Here's the drawing with two shaded views (mm, measured from the low corner). I have some questions. Give positions to 0.01 mm unless a question says otherwise; leave off trailing zeros. Order: outer loops, then holes, each group sorted by start corner. A loop starts at its lowest first (then second) coordinate and runs counter-clockwise, first axis right, second up. Notation, with made-up numbers: M -0.5,86.5 L 43.5,86.5 A14 ccw 43.5,106.5 Z; hole C 22,74.5 d8. An arc over 180 degrees is marked long. Use a Markdown table: item, result. Add a question column.
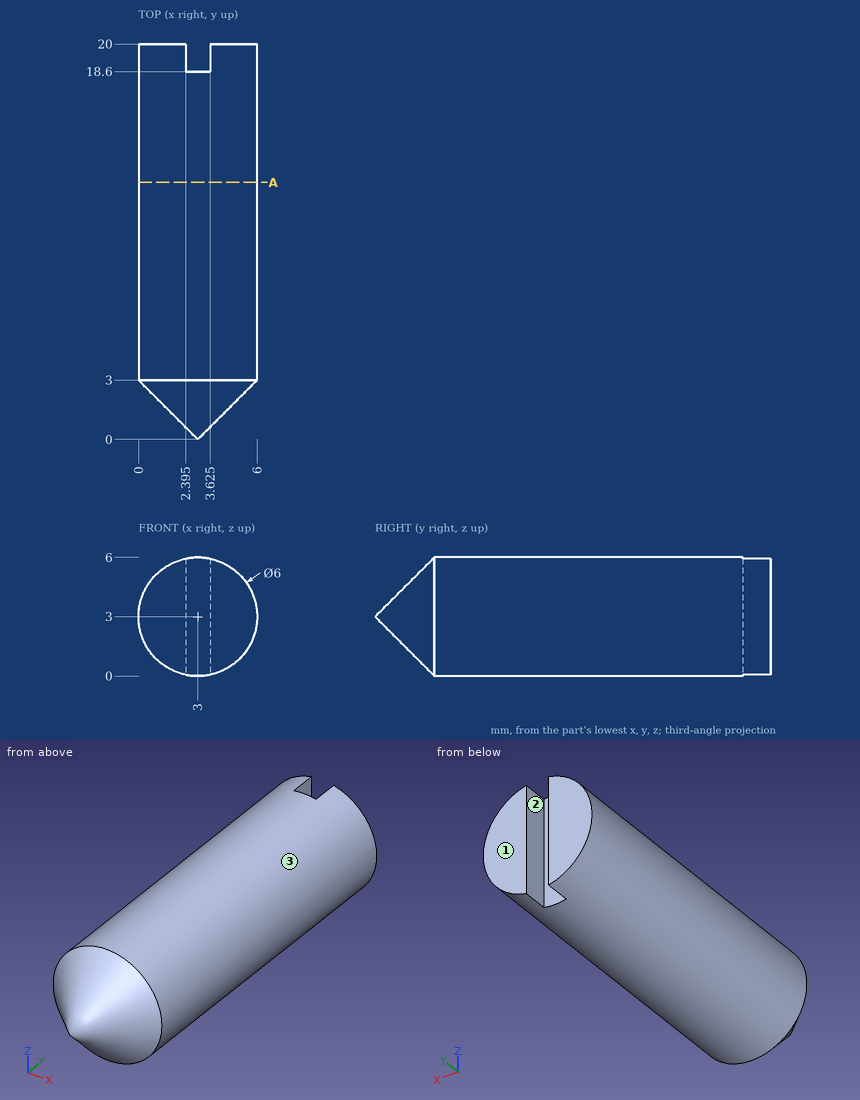
1) Suppose I cut it at A-A on y = 13. Please give me the cut outline in (x, z), and give its area (3 significant figures).
2) We'd pull the mould along X, two halves only. Please class the marked faces 1, 2 and 3: pulls with the +X half, pulls with the -X half, needs draft (parallel to the pull), parting line crosses it, or undercut.
3) Please list where these lines run through material, in increasing order: line 1 (X direction, y = 19, z = 2.1) (3 decimals); line 2 (Z direction, x = 2.9, y = 8.5); line 3 (X direction, y = 14.5, z = 2.2). Write a range as from..to.
4) For pin 1 (1 mm diameter, centred on x = 1, z = 3, fed in from -Y); pin 2 (2 mm diameter, centred on x = 1.5, z = 3, fed in from -Y); pin 3 (1.5 mm diameter, centred on y = 17.5, z = 1.5, fed in from -X), each with a flat end and sliding along its axis, tell me the tip position at first contact or that it passes through.
Values found:
| question | item | result |
|---|---|---|
| 1 | outline | C 3,3 d6 |
| 1 | area | 28.3 mm^2 |
| 2 | face 1 | needs draft |
| 2 | face 2 | undercut |
| 2 | face 3 | parting line crosses it |
| 3 | line 1 | x = 0.138..2.395, 3.625..5.862 |
| 3 | line 2 | z = 0..6 |
| 3 | line 3 | x = 0.11..5.89 |
| 4 | pin 1 | stops at y = 1.5 |
| 4 | pin 2 | stops at y = 0.5 |
| 4 | pin 3 | stops at x = 0.1 |
